from build123d import *

# Parameters (mm, degrees)
BOSS_EXTRUDE1_DEPTH = 6.35
SKETCH2_W           = 27.9781
SKETCH2_H           = 17.4625
BOSS_EXTRUDE2_DEPTH = 6.35


with BuildPart() as part:
    # Sketch1 → Boss-Extrude1 (new body)
    with BuildSketch(Plane(origin=(0, 0, 0), x_dir=(1, 0, 0), z_dir=(0, 1, 0))):
        Polygon((262.669201475, 448.360447089), (367.463251475, 448.360447089), (367.463251475, 430.897947089), (395.441351475, 430.897947089), (395.441351475, 448.360447089), (500.235401475, 448.360447089), (486.227301475, 10.210447089), (384.031988975, 10.210447089), (384.031988975, 230.872947089), (378.872613975, 230.872947089), (378.872613975, 10.210447089), (276.677301475, 10.210447089), align=None)
    extrude(amount=-BOSS_EXTRUDE1_DEPTH)

    # Sketch2 → Boss-Extrude2 (add)
    with BuildSketch(Plane(origin=(0, 0, 0), x_dir=(1, 0, 0), z_dir=(0, 1, 0))):
        with Locations((381.452301475, 439.629197089)):
            Rectangle(SKETCH2_W, SKETCH2_H)
    extrude(amount=-BOSS_EXTRUDE2_DEPTH)


solid = part.part
Geometry check sheet. Reference: the model listing, model coordinates, mm. Round coordinates to 2 decimals unless told otherwise and drop trailing zeros. Loops run counter-clockwise (first coordinate to the right, second up) from the corner with the lowest first, then second, coordinate; pieces in that order, holes last.
Item 1: Cross-section at D-D on z = -325. Record the boundary of the cut face in (x, y), then the cut area to 3 significant figures.
Item 2: Cross-section at C-C on z = -219. Record the boundary of the cut face in (x, y), then the cut area to 3 significant figures.
Item 3: Gauge pin test, flat ends, axial feed: pin 1 (1 mm diameter, centred on y = -5, z = -104.5, fed in from +X); pin 2 (2.5 mm diameter, centred on x = 381.5, y = -2.5, fed in from +Z); pin 3 (3 mm diameter, centred on y = -3.5, z = -142, fed in from -X). Record the tip position at first contact, or that the pin passes through.
Item 4: Thickness scan on line 1 (X direction, y = -5.75, z = -192); line 2 (X direction, y = -3, z = -141); line 3 (X direction, y = -5.5, z = -350.5). Record the ranges inside material, lowest first.
Item 5: Cross-section at A-A on z = -175. Record the boundary of the cut face in (x, y).
Item 6: Cross-section at B-B on y = -4. Record the boundary of the cut face in (x, z), then the cut area to 3 significant figures.
Answer sheet:
1. outline: (266.61, -6.35) - (496.29, -6.35) - (496.29, 0) - (266.61, 0) - close
1. area: 1,460 mm2
2. outline: (270, -6.35) - (378.87, -6.35) - (378.87, 0) - (270, 0) - close; (384.03, -6.35) - (492.9, -6.35) - (492.9, 0) - (384.03, 0) - close
2. area: 1,380 mm2
3. pin 1: stops at x = 489.26
3. pin 2: stops at z = -230.87
3. pin 3: stops at x = 272.42
4. line 1: x = 270.87 to 378.87, 384.03 to 492.04
4. line 2: x = 272.5 to 378.87, 384.03 to 490.41
4. line 3: x = 265.8 to 497.11
5. outline: (271.41, -6.35) - (378.87, -6.35) - (378.87, 0) - (271.41, 0) - close; (384.03, -6.35) - (491.5, -6.35) - (491.5, 0) - (384.03, 0) - close
6. outline: (262.67, -448.36) - (500.24, -448.36) - (486.23, -10.21) - (384.03, -10.21) - (384.03, -230.87) - (378.87, -230.87) - (378.87, -10.21) - (276.68, -10.21) - close
6. area: 96,800 mm2
